Build history of the part. All positions in model axes, mm. Face numbers are marked on the shaded views. A direction names the side the tool comes from. Coordinates: 2 decimals unless noted, no trailing zeros. Write each loop counter-clockwise with the first axis right and the second up, starting at its lowest first coordinate (ties: lowest second). Pieces come first, ordered by that corner, then holes.
```python
from build123d import *

# Parameters (mm, degrees)
BOSS_EXTRUDE1_DEPTH = 8.6
SKETCH5_W           = 8.5
SKETCH5_H           = 23.85
CUT_EXTRUDE3_DEPTH  = 10
SKETCH6_W           = 15.85
SKETCH6_H           = 4.6
CUT_EXTRUDE4_DEPTH  = 10
SKETCH7_W           = 15.85
SKETCH7_H           = 4.6
CUT_EXTRUDE5_DEPTH  = 10
SKETCH9_W           = 7
SKETCH9_H           = 7
BOSS_EXTRUDE3_DEPTH = 3
SKETCH10_R          = 1.5
CUT_EXTRUDE6_DEPTH  = 3


with BuildPart() as part:
    # Sketch1 → Boss-Extrude1 (new body)
    with BuildSketch(Plane(origin=(0, 0, 0), x_dir=(1, 0, 0), z_dir=(0, 1, 0))):
        Polygon((-10.5, 0), (-10.5, -24.849623113), (-10.5, -29.849623113), (7.5, -29.849623113), (10.5, -29.849623113), (10.5, -24.849623113), (10.5, 0), align=None)
    extrude(amount=BOSS_EXTRUDE1_DEPTH)

    # Sketch5 → Cut-Extrude3 (cut)
    with BuildSketch(Plane(origin=(0, 8.6, 0), x_dir=(1, 0, 0), z_dir=(0, 1, 0))):
        with Locations((0, -14.924623113)):
            Rectangle(SKETCH5_W, SKETCH5_H)
    extrude(amount=-CUT_EXTRUDE3_DEPTH, mode=Mode.SUBTRACT)

    # Sketch6 → Cut-Extrude4 (cut)
    with BuildSketch(Plane.ZY.offset(10.5)):
        with Locations((14.925, 4.3)):
            Rectangle(SKETCH6_W, SKETCH6_H)
    extrude(amount=-CUT_EXTRUDE4_DEPTH, mode=Mode.SUBTRACT)

    # Sketch7 → Cut-Extrude5 (cut)
    with BuildSketch(Plane(origin=(10.5, 0, 0), x_dir=(0, 0, -1), z_dir=(1, 0, 0))):
        with Locations((-14.924623113, 4.3)):
            Rectangle(SKETCH7_W, SKETCH7_H)
    extrude(amount=-CUT_EXTRUDE5_DEPTH, mode=Mode.SUBTRACT)

    # Sketch9 → Boss-Extrude3 (add)
    with BuildSketch(Plane.XZ):
        with Locations((-14, 26.349623113)):
            Rectangle(SKETCH9_W, SKETCH9_H)
        with Locations((14, 26.349623113)):
            Rectangle(SKETCH9_W, SKETCH9_H)
        with Locations((-14, 3.5)):
            Rectangle(SKETCH9_W, SKETCH9_H)
        with Locations((14, 3.5)):
            Rectangle(SKETCH9_W, SKETCH9_H)
    extrude(amount=-BOSS_EXTRUDE3_DEPTH)

    # Sketch10 → Cut-Extrude6 (cut)
    with BuildSketch(Plane(origin=(0, 3, 0), x_dir=(1, 0, 0), z_dir=(0, 1, 0))):
        with Locations(Location((-13.5, -3.5, 0), (0, 0, 270))):
            Circle(SKETCH10_R)
        with Locations(Location((-13.5, -26.349623113, 0), (0, 0, 270))):
            Circle(SKETCH10_R)
        with Locations(Location((13.5, -26.349623113, 0), (0, 0, 90))):
            Circle(SKETCH10_R)
        with Locations(Location((13.5, -3.5, 0), (0, 0, 90))):
            Circle(SKETCH10_R)
    extrude(amount=-CUT_EXTRUDE6_DEPTH, mode=Mode.SUBTRACT)


solid = part.part
```
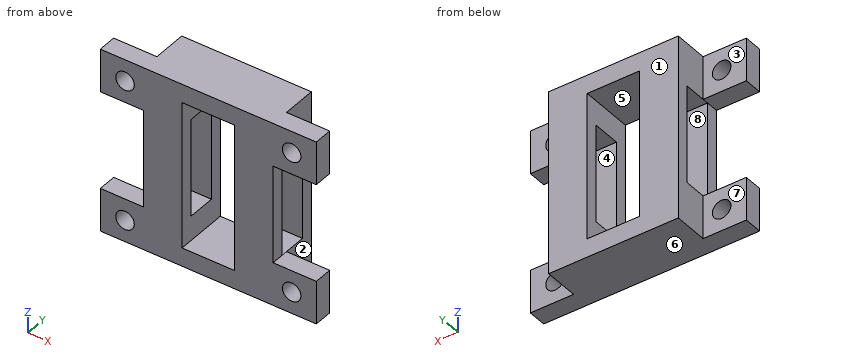
1. Saw through at D-D on x = 13.5. List the corners of the cut face in (y, z), plus the area to 3 significant figures.
Computed values:
outline: (0, 0) - (3, 0) - (3, 2) - (0, 2) - close; (0, 5) - (3, 5) - (3, 7) - (0, 7) - close; (0, 22.85) - (3, 22.85) - (3, 24.85) - (0, 24.85) - close; (0, 27.85) - (3, 27.85) - (3, 29.85) - (0, 29.85) - close
area: 24.0 mm2
2. Probe line 1 along X through (y, z) = (1.4, 3.5); line 2 along Z through (x, y) = (13.5, 1.75); line 3 along Y through (x, z) = (-9, 20). List the from-to ranges inside material, lowest first.
Computed values:
line 1: x = -17.5 to -15, -12 to -4.25, 4.25 to 12, 15 to 17.5
line 2: z = 0 to 2, 5 to 7, 22.85 to 24.85, 27.85 to 29.85
line 3: y = 0 to 2, 6.6 to 8.6
3. Mould opens along Z. For the marked faces 6, 7 and 8 say: +Z half, -Z half, draft (parallel to the pull), parting line (faces both ways), or undercut.
Computed values:
face 6: -Z half
face 7: draft
face 8: undercut
4. Saw through at B-B on z = 3.5. List the corners of the cut face in (x, y), plus the area to 4 significant figures.
Computed values:
outline: (-17.5, 0) - (-15, 0) - (-15, 3) - (-17.5, 3) - close; (-12, 0) - (-4.25, 0) - (-4.25, 8.6) - (-10.5, 8.6) - (-10.5, 3) - (-12, 3) - close; (4.25, 0) - (12, 0) - (12, 3) - (10.5, 3) - (10.5, 8.6) - (4.25, 8.6) - close; (15, 0) - (17.5, 0) - (17.5, 3) - (15, 3) - close
area: 131.5 mm2
5. 3-axis set-ups, long thin cutter, end or side, ignore diameter. For the marked faces 1, 2, 3, 4 and 5: which of +Z, -Z, +X, -X, +Y, -Y reach the whole face in a straight line?
Computed values:
face 1: +Z, -Z, +X, -X, +Y
face 2: +Z, -Z, +X, +Y
face 3: +Z, -Z, -X, +Y
face 4: +X, -X
face 5: +Y, -Y
6. Saw through at C-C on y = 1.5. List the corners of the cut face in (x, z), plus the area to 3 significant figures.
Computed values:
outline: (-17.5, 0) - (17.5, 0) - (17.5, 7) - (10.5, 7) - (10.5, 22.85) - (17.5, 22.85) - (17.5, 29.85) - (-17.5, 29.85) - (-17.5, 22.85) - (-10.5, 22.85) - (-10.5, 7) - (-17.5, 7) - close; hole circle Ø3 at (-13.5, 3.5); hole circle Ø3 at (-13.5, 26.35); hole (-4.25, 3) - (4.25, 3) - (4.25, 26.85) - (-4.25, 26.85) - close; hole circle Ø3 at (13.5, 3.5); hole circle Ø3 at (13.5, 26.35)
area: 592 mm2
7. Flat gauge pins, fed straight in: pin 1 (3.5 mm diameter, centred on x = -13.5, z = 5, fed in from +Y); pin 2 (0.6 mm diameter, centred on y = 1.5, z = 16, fed in from +X). Where does each tip first touch, or does it go through?
Computed values:
pin 1: stops at y = 3
pin 2: stops at x = 10.5
8. Saw through at A-A on x = 1. List the corners of the cut face in (y, z).
Computed values:
outline: (0, 0) - (8.6, 0) - (8.6, 3) - (0, 3) - close; (0, 26.85) - (8.6, 26.85) - (8.6, 29.85) - (0, 29.85) - close
